Verification items for the finished model (mm, model axes). A direction names the side the tool comes from. Give positions to 0.01 mm unless a question says otherwise; leave off trailing zeros. Loops run counter-clockwise (first coordinate to the right, second up) from the corner with the lowest first, then second, coordinate; pieces in that order, holes last. Notation, with made-up numbers: (29.5, 61) - (47.5, 61) arc R10 cw to (47.5, 80) - close; hole circle Ø4 at (58, 83). An arc over 180 degrees is marked (long way). Put each result on its own line as item: value. Start each with the question number.
```python
from build123d import *

# Parameters (mm, degrees)
SKETCH_W     = 30
SKETCH_H     = 25
PAD_DEPTH    = 2
FILLET_R     = 10
FILLET001_R  = 10
PAD001_DEPTH = 40
FILLET002_R  = 10
FILLET003_R  = 10
PAD002_DEPTH = 2
FILLET004_R  = 5
FILLET005_R  = 5
SKETCH003_R  = 2
POCKET_DEPTH = 5


with BuildPart() as part:
    # Sketch → Pad (new body)
    with BuildSketch(Plane.XY):
        with Locations((15, -12.5)):
            Rectangle(SKETCH_W, SKETCH_H)
    extrude(amount=PAD_DEPTH)

    # Fillet
    fillet_edges = [part.edges().sort_by_distance(p)[0] for p in [
        (0, -25, 1),
    ]]
    fillet(fillet_edges, radius=FILLET_R)

    # Fillet001
    fillet001_edges = [part.edges().sort_by_distance(p)[0] for p in [
        (30, -25, 1),
    ]]
    fillet(fillet001_edges, radius=FILLET001_R)

    # Sketch001 (on Face5 of Fillet001) → Pad001 (join)
    with BuildSketch(Plane.XY.offset(2)):
        with BuildLine():
            ThreePointArc((30, -10.46031), (15, -5), (0, -10.46031))
            Line((0, -12.46031), (0, -10.46031))
            ThreePointArc((30, -12.46031), (15, -7), (0, -12.46031))
            Line((30, -12.46031), (30, -10.46031))
        make_face()
    extrude(amount=PAD001_DEPTH)

    # Fillet002
    fillet002_edges = [part.edges().sort_by_distance(p)[0] for p in [
        (0, 0, 1),
    ]]
    fillet(fillet002_edges, radius=FILLET002_R)

    # Fillet003
    fillet003_edges = [part.edges().sort_by_distance(p)[0] for p in [
        (30, 0, 1),
    ]]
    fillet(fillet003_edges, radius=FILLET003_R)

    # Sketch002 (on Face16 of Fillet003) → Pad002 (join)
    with BuildSketch(Plane.XY.offset(42)):
        with BuildLine():
            ThreePointArc((30, -12.459868), (15, -7), (0, -12.459868))
            Line((0, -12.459868), (0, -5.459868))
            ThreePointArc((30, -5.459868), (15, 0), (0, -5.459868))
            Line((30, -12.459868), (30, -5.459868))
        make_face()
    extrude(amount=PAD002_DEPTH)

    # Fillet004
    fillet004_edges = [part.edges().sort_by_distance(p)[0] for p in [
        (0, -5.459868, 43),
    ]]
    fillet(fillet004_edges, radius=FILLET004_R)

    # Fillet005
    fillet005_edges = [part.edges().sort_by_distance(p)[0] for p in [
        (30, -5.459868, 43),
    ]]
    fillet(fillet005_edges, radius=FILLET005_R)

    # Sketch003 (on Face21 of Fillet005) → Pocket (cut)
    with BuildSketch(Plane.XY.offset(2)):
        with Locations((7.5, -16)):
            Circle(SKETCH003_R)
        with Locations((22.5, -16)):
            Circle(SKETCH003_R)
    extrude(amount=-POCKET_DEPTH, mode=Mode.SUBTRACT)


solid = part.part
```
1) Set-up check for faces 1 (the face through (15, -7, 22)), 2 (the face through (15, -4, 42)), 3 (the face through (2.85, -3.01, 1.01)), 4 (the face through (15, 0, 1)), 5 (the face through (26.99, -2.85, 1.01)): record each of +Z, -Z, +X, -X, +Y, -Y from which the full face is reachable in a straight line by a thin tool's end or side.
2) Section check C-C, the plane z = 17. Enter the section's corners in (x, y).
3) Scan lines: line 1 along Z through (x, y) = (18.5, -19); line 2 along Y through (x, z) = (7.5, 1.65); line 3 along Y through (x, z) = (7.75, 41.5). Record each from-to range of solid material in increasing order. Write a range as from..to.
4) Depth check by flat-ended pin: P1, Ø6.5, axis at x = 7.5, y = -16, coming from the +Z side; P2, Ø2, axis at y = -3.5, z = 13, coming from the -X side; P3, Ø6, axis at x = 19, z = 19, coming from the +Y side; P4, Ø12, axis at x = 3.5, z = 17, coming from the +Y side. Enter the tip coordinate at first touch or a pass-through.
5) Section check B-B, the plane y = -16. Enter the section's corners in (x, z), plus the area to 3 significant figures.
6) Draft check along Z on faces 6 (the face through (0, -11, 20)), 7 (the face through (15, -16, 2)), 8 (the face through (15, -4, 2)), 9 (the face through (15, -5, 22)). Enter one of: pulls with the +Z half, pulls with the -Z half, needs draft (parallel to the pull), parting line crosses it, or undercut.
Results are:
1. face 1: +Z, -Y
1. face 2: +Y
1. face 3: -Z, -X, +Y
1. face 4: +Z, -Z, +X, -X, +Y
1. face 5: -Z, +X, +Y
2. outline: (0, -12.46) arc R23.33 cw to (30, -12.46) - (30, -10.46) arc R23.33 ccw to (0, -10.46) - close
3. line 1: z = 0..2
3. line 2: y = -24.68..-18, -14..-0.32
3. line 3: y = -8.15..-6.15
4. P1: stops at z = 2
4. P2: passes through
4. P3: stops at y = -5.02
4. P4: stops at y = -5.66
5. outline: (0.05, 0) - (5.5, 0) - (5.5, 2) - (0.05, 2) - close; (9.5, 0) - (20.5, 0) - (20.5, 2) - (9.5, 2) - close; (24.5, 0) - (29.95, 0) - (29.95, 2) - (24.5, 2) - close
5. area: 43.8 mm2
6. face 6: needs draft
6. face 7: pulls with the +Z half
6. face 8: undercut
6. face 9: undercut
